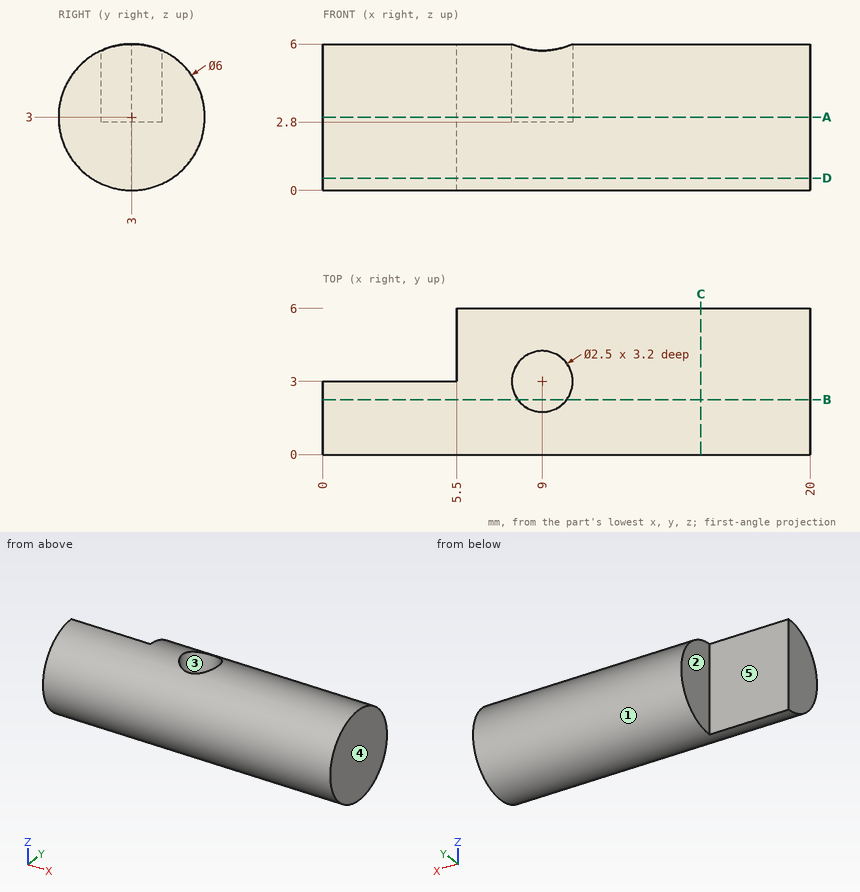
Job drawing, mm, ordinate dimensions from the low corner. One solid piece. A direction names the side the tool comes from. Give positions to 0.01 mm unless a question says otherwise; leave off trailing zeros. Write each loop counter-clockwise with the first axis right and the second up, starting at its lowest first coordinate (ties: lowest second). Pieces come first, ordered by that corner, then holes. Notation, with made-up numbers: M 83,5 L 87,5 A17 ccw 87,11 Z; hole C -27,78 d9. An arc over 180 degrees is marked long. Put each result on its own line as item: value. Start each with the question number.
(1) Probe L1, parallel to Y at x = 9, z = 3.9; L2, parallel to Y at x = 9, z = 5.25; L3, parallel to X at y = 4.75, z = 1. List the from-to ranges inside material, lowest first.
(2) Which spindle directions (+Z, -Z, +X, -X, +Y, -Y) get a long thin tool onto all of the face, cutting with end or side? Do the marked faces 1 and 2. Say none if no direction does.
(3) Flat gauge pins, fed straight in: pin 1 Ø1 at (x, z) = (3, 5) entering from -Y; pin 2 Ø1 at (x, z) = (15.5, 2) entering from -Y; pin 3 Ø1.7 at (x, z) = (3.5, 4.5) entering from +Y. Where does each tip first touch, or does it go through?
(4) Band-saw the part on A-A, the plane z = 3. Write the cut outline in (x, y).
(5) Mould opens along X. For the marked faces 3, 4 and 5 say: +X half, -X half, draft (parallel to the pull), parting line (faces both ways), or undercut.
(6) Band-saw the part on B-B, the plane y = 2.25. Write the cut outline in (x, z), and give its area (3 significant figures).
(7) Band-saw the part on D-D, the plane z = 0.5. Write the cut outline in (x, y).
(8) Band-saw the part on C-C, the plane x = 15.5. Write the cut outline in (y, z).
Response values:
1. L1: y = 0.14 to 1.75, 4.25 to 5.86
1. L2: y = 1.02 to 1.75, 4.25 to 4.98
1. L3: x = 5.5 to 20
2. face 1: +X, -X
2. face 2: +Z, -Z, -X, +Y
3. pin 1: stops at y = 0.4
3. pin 2: stops at y = 0.04
3. pin 3: stops at y = 3
4. outline: M 0,0 L 20,0 L 20,6 L 5.5,6 L 5.5,3 L 0,3 Z; hole C 9,3 d2.5
5. face 3: undercut
5. face 4: +X half
5. face 5: draft
6. outline: M 0,0.1 L 20,0.1 L 20,5.9 L 10,5.9 L 10,2.8 L 8,2.8 L 8,5.9 L 0,5.9 Z
6. area: 110 mm2
7. outline: M 0,1.34 L 20,1.34 L 20,4.66 L 5.5,4.66 L 5.5,3 L 0,3 Z
8. outline: C 3,3 d6
